Could you check a few things on this drawing? It's one solid part, dimensions in mm from its lowest x, y, z. A direction names the side the tool comes from. Round coordinates to 2 decimals unless told otherwise and drop trailing zeros. Write each loop counter-clockwise with the first axis right and the second up, starting at its lowest first coordinate (ties: lowest second). Pieces come first, ordered by that corner, then holes. Notation, with made-up numbers: (-3.5, 63) -> (45.5, 63) arc R18 cw to (45.5, 67) -> close; hole circle Ø2 at (84, 77.25). An arc over 180 degrees is marked (long way). Answer in a Markdown table with one row per item.
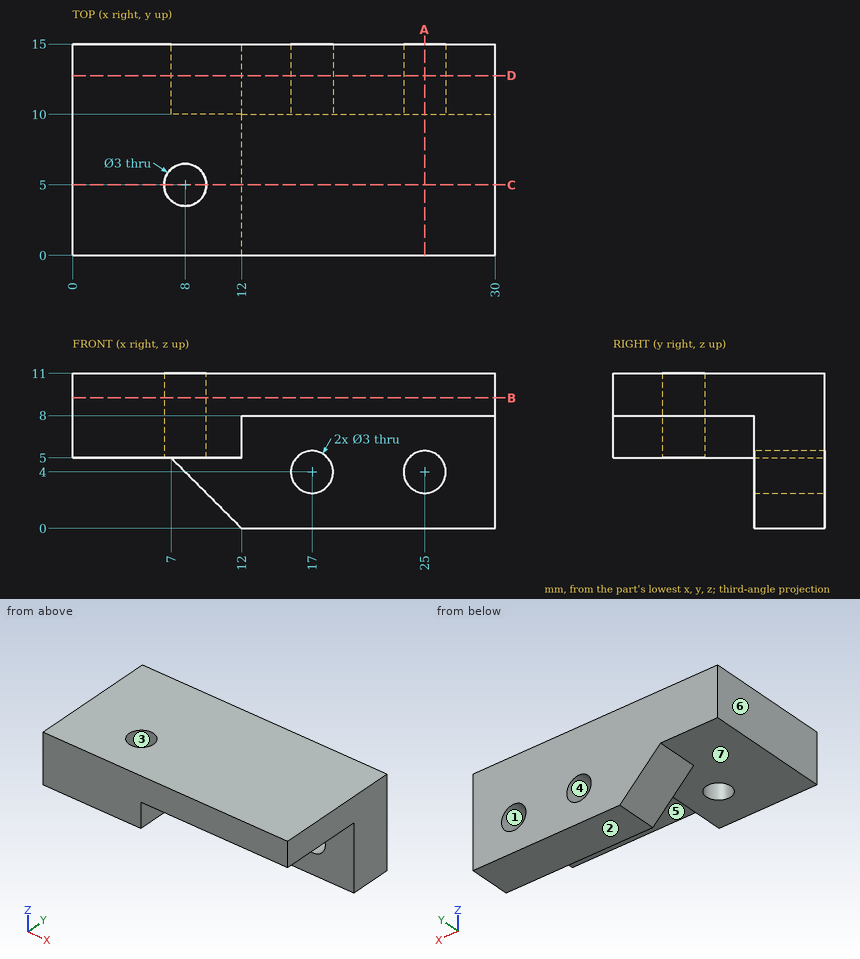
1) I want a section at B-B, the plane z = 9.25. List the corners of the cut face in (x, y) for me.
Response:
| item | result |
|---|---|
| outline | (0, 0) -> (30, 0) -> (30, 15) -> (0, 15) -> close; hole circle Ø3 at (8, 5) |
2) Which directions (+Z, -Z, +X, -X, +Y, -Y) give clear straight access to the entire face, cutting with the end or side of a thin tool? Please do the marked faces 5, 6 and 7.
Response:
| item | result |
|---|---|
| face 5 | -Z, +X, -Y |
| face 6 | +Z, -Z, -X, +Y, -Y |
| face 7 | -Z, -X, -Y |
3) I want a section at C-C, the plane y = 5. List the corners of the cut face in (x, z) for me, and give its area (3 significant figures).
Response:
| item | result |
|---|---|
| outline | (0, 5) -> (6.5, 5) -> (6.5, 11) -> (0, 11) -> close; (9.5, 5) -> (12, 5) -> (12, 8) -> (30, 8) -> (30, 11) -> (9.5, 11) -> close |
| area | 108 mm^2 |
4) I want a section at D-D, the plane y = 12.75. Count the separate pieces of the cut face and the enclosed holes in it, and give its area (3 significant figures).
Response:
| item | result |
|---|---|
| separate pieces | 1 |
| enclosed holes | 2 |
| area | 268 mm^2 |
5) I need wall thicknesses on line 1 (X direction, y = 11.3, z = 4); line 2 (X direction, y = 5, z = 8.55); line 3 (X direction, y = 10.5, z = 4.25). Which ranges of each line are inside material? Lowest first, please. Write a range as [from, to].
Response:
| item | result |
|---|---|
| line 1 | x = [8, 15.5], [18.5, 23.5], [26.5, 30] |
| line 2 | x = [0, 6.5], [9.5, 30] |
| line 3 | x = [7.75, 15.52], [18.48, 23.52], [26.48, 30] |
6) I want a section at A-A, the plane x = 25. List the corners of the cut face in (y, z) for me, and give its area (3 significant figures).
Response:
| item | result |
|---|---|
| outline | (0, 8) -> (10, 8) -> (10, 5.5) -> (15, 5.5) -> (15, 11) -> (0, 11) -> close; (10, 0) -> (15, 0) -> (15, 2.5) -> (10, 2.5) -> close |
| area | 70.0 mm^2 |
7) We'd pull the mould along Z, two halves only. Please class the marked faces 1, 2, 3 and 4: +Z half, -Z half, draft (parallel to the pull), parting line (faces both ways), or undercut.
Response:
| item | result |
|---|---|
| face 1 | undercut |
| face 2 | -Z half |
| face 3 | draft |
| face 4 | undercut |
8) For pin 1 (4 mm diameter, centred on x = 8, y = 5, fed in from -Z); pin 2 (1.5 mm diameter, centred on y = 4, z = 6.5, fed in from +X); pin 3 (4 mm diameter, centred on x = 16, z = 2, fed in from -Y), each with a flat end and sliding along its axis, tell me the tip position at first contact or that it passes through.
Response:
| item | result |
|---|---|
| pin 1 | stops at z = 5 |
| pin 2 | stops at x = 12 |
| pin 3 | stops at y = 10 |
